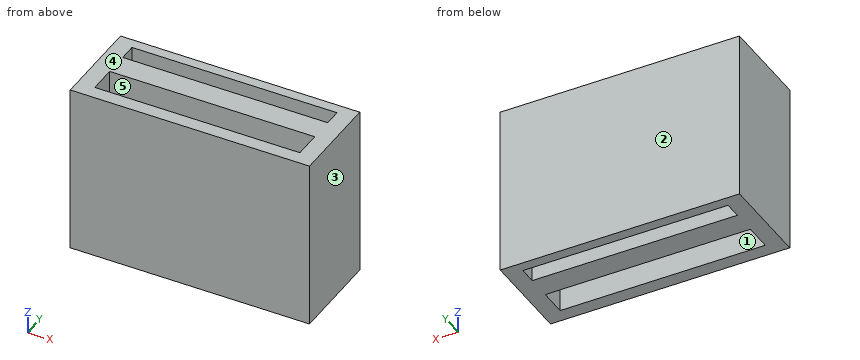
```python
from build123d import *

# Parameters (mm, degrees)
SKETCH2_W           = 70
SKETCH2_H           = 27
SKETCH2_W_2         = 60
SKETCH2_H_2         = 8
SKETCH2_H_3         = 5
BOSS_EXTRUDE1_DEPTH = 50


with BuildPart() as part:
    # Sketch2 → Boss-Extrude1 (new body)
    with BuildSketch(Plane.XY):
        with Locations((35, 13.5)):
            Rectangle(SKETCH2_W, SKETCH2_H)
        with Locations((35, 8)):
            Rectangle(SKETCH2_W_2, SKETCH2_H_2, mode=Mode.SUBTRACT)
        with Locations((35, 21.5)):
            Rectangle(SKETCH2_W_2, SKETCH2_H_3, mode=Mode.SUBTRACT)
    extrude(amount=BOSS_EXTRUDE1_DEPTH)


solid = part.part
```
For this review, take the finished solid that the model builds, in its own axes (mm). Face numbers are marked on the shaded views. A direction names the side the tool comes from. Give positions to 0.01 mm unless a question says otherwise; leave off trailing zeros. Loops run counter-clockwise (first coordinate to the right, second up) from the corner with the lowest first, then second, coordinate; pieces in that order, holes last. Notation, with made-up numbers: M 65,70.5 L 84,70.5 A10 cw 84,87.5 Z; hole C -35.5,-20 d6. An arc over 180 degrees is marked long. One line per item, written item: value. Start each with the question number.
Q1. Add section A-A (y = 10.5). Give the boundary of the cut face in (x, z), and give its area (3 significant figures).
Q2. For L1, parallel to Y at x = 24, z = 3.5; L2, parallel to X at y = 19.5, z = 10.5, list the stretches that pass through material, from the lowest coordinate up.
Q3. Draft analysis for pull direction Y (two halves, no side actions). For the marked faces 1, 2 and 3, state which applies: released by +Y, released by -Y, zero draft, split by the parting line, or undercut.
Q4. Add section B-B (z = 13.5). Give the boundary of the cut face in (x, y), and give its area (3 significant figures).
Q5. Add section C-C (x = 29.5). Give the boundary of the cut face in (y, z), and give its area (3 significant figures).
Q6. Machinability: for the marked faces 4 and 5, which of the approach directions +Z, -Z, +X, -X, +Y, -Y give a long, thin tool a straight path to every point of the face, cutting with its end or side? Answer none if there is none.
Reply:
1. outline: M 0,0 L 5,0 L 5,50 L 0,50 Z; M 65,0 L 70,0 L 70,50 L 65,50 Z
1. area: 500 mm²
2. L1: 0 to 4, 12 to 19, 24 to 27
2. L2: 0 to 5, 65 to 70
3. face 1: undercut
3. face 2: released by +Y
3. face 3: zero draft
4. outline: M 0,0 L 70,0 L 70,27 L 0,27 Z; hole M 5,4 L 65,4 L 65,12 L 5,12 Z; hole M 5,19 L 65,19 L 65,24 L 5,24 Z
4. area: 1,110 mm²
5. outline: M 0,0 L 4,0 L 4,50 L 0,50 Z; M 12,0 L 19,0 L 19,50 L 12,50 Z; M 24,0 L 27,0 L 27,50 L 24,50 Z
5. area: 700 mm²
6. face 4: +Z, +X, -X, +Y, -Y
6. face 5: +Z, -Z
